Drawing for the job (mm, zero at the part's lowest x, y, z). A direction names the side the tool comes from. Round coordinates to 2 decimals unless told otherwise and drop trailing zeros. Order: outer loops, then holes, each group sorted by start corner. A loop starts at its lowest first (then second) coordinate and runs counter-clockwise, first axis right, second up. Notation, with made-up numbers: (67, 4.25) - (82, 4.25) arc R11 ccw to (82, 14.25) - close; hole circle Ø11 at (-9, 81). An arc over 180 degrees is marked (long way). Put each result on its own line as item: value. Start each with the question number.
Item 1: Mould opens along X. For the marked faces 1, 2 and 3 say: pulls with the +X half, pulls with the -X half, needs draft (parallel to the pull), parting line crosses it, or undercut.
Item 2: Saw through at A-A on z = 4.25. List the corners of the cut face in (x, y).
Item 3: Probe probe 1 along X at (y, z) = (6.5, 1.75); probe 2 along X at (y, z) = (28.5, 1.25); probe 3 along X at (y, z) = (23.5, 7). List the from-to ranges inside material, lowest first.
Item 4: Which spindle directions (+Z, -Z, +X, -X, +Y, -Y) get a long thin tool onto all of the face, cutting with end or side? Do the marked faces 4, 5, 6, 7 and 8. Say none if no direction does.
Item 5: Saw through at D-D on y = 20.5. List the corners of the cut face in (x, z).
Item 6: Saw through at C-C on x = 4.5. List the corners of the cut face in (y, z), plus the area to 3 significant figures.
Item 7: Saw through at B-B on y = 16. List the corners of the cut face in (x, z), plus the area to 3 significant figures.
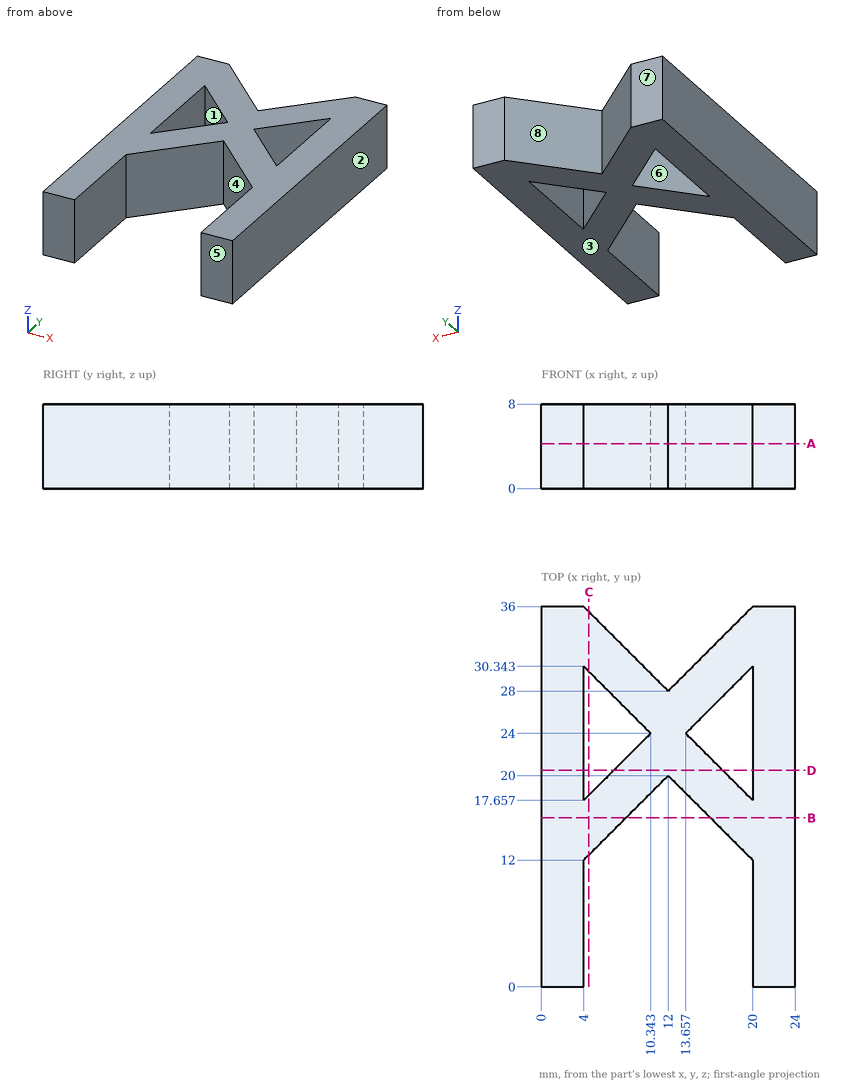
Results found:
1. face 1: undercut
1. face 2: pulls with the +X half
1. face 3: needs draft
2. outline: (0, 0) - (4, 0) - (4, 12) - (12, 20) - (20, 12) - (20, 0) - (24, 0) - (24, 36) - (20, 36) - (12, 28) - (4, 36) - (0, 36) - close; hole (4, 17.66) - (10.34, 24) - (4, 30.34) - close; hole (13.66, 24) - (20, 17.66) - (20, 30.34) - close
3. probe 1: x = 0 to 4, 20 to 24
3. probe 2: x = 0 to 4, 5.84 to 11.5, 12.5 to 18.16, 20 to 24
3. probe 3: x = 0 to 4, 9.84 to 14.16, 20 to 24
4. face 4: +Z, -Z, -Y
4. face 5: +Z, -Z, +X, -X, -Y
4. face 6: +Z, -Z
4. face 7: +Z, -Z, +X, -X, +Y
4. face 8: +Z, -Z, +Y
5. outline: (0, 0) - (4, 0) - (4, 8) - (0, 8) - close; (6.84, 0) - (17.16, 0) - (17.16, 8) - (6.84, 8) - close; (20, 0) - (24, 0) - (24, 8) - (20, 8) - close
6. outline: (12.5, 0) - (18.16, 0) - (18.16, 8) - (12.5, 8) - close; (29.84, 0) - (35.5, 0) - (35.5, 8) - (29.84, 8) - close
6. area: 90.5 mm²
7. outline: (0, 0) - (8, 0) - (8, 8) - (0, 8) - close; (16, 0) - (24, 0) - (24, 8) - (16, 8) - close
7. area: 128 mm²
